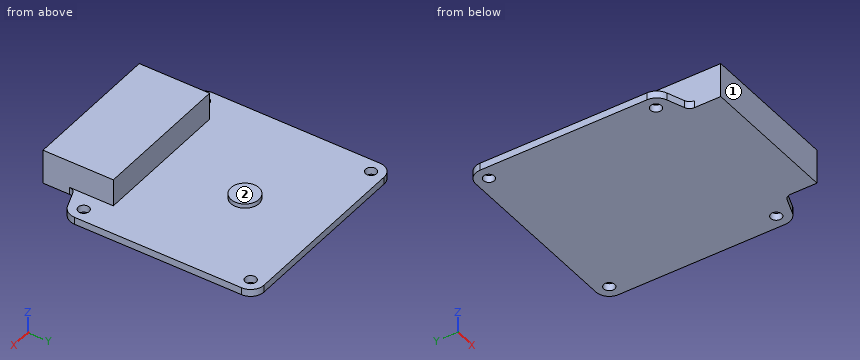
```python
from build123d import *

# Parameters (mm, degrees)
SKETCH1_R           = 3.2
SKETCH1_R_2         = 1.25
BOSS_EXTRUDE1_DEPTH = 1.65
SKETCH2_W           = 32
SKETCH2_H           = 16
BOSS_EXTRUDE2_DEPTH = 6.2
SKETCH1_2_R         = 3.2
BOSS_EXTRUDE3_DEPTH = 2.65


with BuildPart() as part:
    # Sketch1 → Boss-Extrude1 (new body)
    with BuildSketch(Plane.XY):
        with BuildLine():
            Line((-20, 18), (20, 18))
            ThreePointArc((20, 18), (22.121320344, 17.121320344), (23, 15))
            Line((23, 15), (23, -23))
            ThreePointArc((23, -23), (22.416236427, -24.864680631), (20.873373788, -26.063592072))
            Line((20.873373788, -26.063592072), (17.047054496, -27.491625922))
            ThreePointArc((17.047054496, -27.491625922), (16.287418762, -28.081915652), (16, -29))
            Line((16, -29), (16, -35))
            Line((16, -35), (-16, -35))
            Line((-16, -35), (-16, -29))
            ThreePointArc((-16, -29), (-16.287418762, -28.081915652), (-17.047054496, -27.491625922))
            Line((-17.047054496, -27.491625922), (-20.873373788, -26.063592072))
            ThreePointArc((-20.873373788, -26.063592072), (-22.416236427, -24.864680631), (-23, -23))
            Line((-23, -23), (-23, 15))
            ThreePointArc((-23, 15), (-22.121320344, 17.121320344), (-20, 18))
        make_face()
        Circle(SKETCH1_R, mode=Mode.SUBTRACT)
        with Locations((20, 15)):
            Circle(SKETCH1_R_2, mode=Mode.SUBTRACT)
        with Locations((-20, 15)):
            Circle(SKETCH1_R_2, mode=Mode.SUBTRACT)
        with Locations((-20, -23)):
            Circle(SKETCH1_R_2, mode=Mode.SUBTRACT)
        with Locations((20, -23)):
            Circle(SKETCH1_R_2, mode=Mode.SUBTRACT)
    extrude(amount=BOSS_EXTRUDE1_DEPTH)

    # Sketch2 → Boss-Extrude2 (add)
    with BuildSketch(Plane.XY.offset(1.65)):
        with Locations((0, -27)):
            Rectangle(SKETCH2_W, SKETCH2_H)
    extrude(amount=BOSS_EXTRUDE2_DEPTH)

    # Sketch1<2> → Boss-Extrude3 (add)
    with BuildSketch(Plane.XY):
        Circle(SKETCH1_2_R)
    extrude(amount=BOSS_EXTRUDE3_DEPTH)


solid = part.part
```
Build history of the part. All positions in model axes, mm. Face numbers are marked on the shaded views. A direction names the side the tool comes from. Give positions to 0.01 mm unless a question says otherwise; leave off trailing zeros. Loops run counter-clockwise (first coordinate to the right, second up) from the corner with the lowest first, then second, coordinate; pieces in that order, holes last.
1) Drop flat-ended pins along their axis: P1, Ø4, axis at y = 6, z = 5.5, coming from the +X side; P2, Ø10, axis at x = 5.5, y = -0.5, coming from the +Z side; P3, Ø4, axis at y = -27, z = 3, coming from the +X side; P4, Ø3, axis at x = -20, y = -23, coming from the +Z side. Give the stop position or say it passes through.
Values follow:
P1: passes through
P2: stops at z = 2.65
P3: stops at x = 21.81
P4: stops at z = 1.65
2) 3-axis set-ups, long thin cutter, end or side, ignore diameter. For the marked faces 1 and 2: which of +Z, -Z, +X, -X, +Y, -Y reach the whole face in a straight line?
Values follow:
face 1: +Z, -Z, +X, -X, -Y
face 2: +Z, +X, -X, +Y
3) Band-saw the part on B-B on x = 0. List the corners of the cut face in (y, z).
Values follow:
outline: (-35, 0) - (18, 0) - (18, 1.65) - (3.2, 1.65) - (3.2, 2.65) - (-3.2, 2.65) - (-3.2, 1.65) - (-19, 1.65) - (-19, 7.85) - (-35, 7.85) - close
4) Band-saw the part on C-C on y = 0. List the corners of the cut face in (x, z), then the cut area to 3 significant figures.
Values follow:
outline: (-23, 0) - (23, 0) - (23, 1.65) - (3.2, 1.65) - (3.2, 2.65) - (-3.2, 2.65) - (-3.2, 1.65) - (-23, 1.65) - close
area: 82.3 mm2
5) Band-saw the part on D-D on z = 6. List the corners of the cut face in (x, y).
Values follow:
outline: (-16, -35) - (16, -35) - (16, -19) - (-16, -19) - close
6) Probe line 1 along Y through (x, z) = (20, 0.5); line 2 along Z through (x, y) = (3, 16); line 3 along X through (y, z) = (16, 1). List the from-to ranges inside material, lowest first.
Values follow:
line 1: y = -26.39 to -24.25, -21.75 to 13.75, 16.25 to 18
line 2: z = 0 to 1.65
line 3: x = -22.83 to -20.75, -19.25 to 19.25, 20.75 to 22.83
7) Band-saw the part on A-A on z = 1. List the corners of the cut face in (x, y).
Values follow:
outline: (-23, -23) arc R3.27 ccw to (-20.87, -26.06) - (-17.05, -27.49) arc R1.61 cw to (-16, -29) - (-16, -35) - (16, -35) - (16, -29) arc R1.61 cw to (17.05, -27.49) - (20.87, -26.06) arc R3.27 ccw to (23, -23) - (23, 15) arc R3 ccw to (20, 18) - (-20, 18) arc R3 ccw to (-23, 15) - close; hole circle Ø2.5 at (-20, -23); hole circle Ø2.5 at (-20, 15); hole circle Ø2.5 at (20, -23); hole circle Ø2.5 at (20, 15)
